Autodesk Inventor part; units mm, degrees
ref_plane "YZ Plane" through (0, 0, 0) normal (1, 0, 0) x (0, 1, 0)
ref_plane "XZ Plane" through (0, 0, 0) normal (0, 1, 0) x (-1, 0, 0)
ref_plane "XY Plane" through (0, 0, 0) normal (0, 0, 1) x (1, 0, 0)
sketch "Sketch1" plane through (0, 0, 0) normal (0, 0, 1) x (1, 0, 0)
  point P0 (0, 0)
sketch "Sketch2" plane through (0, 0, 0) normal (0, 0, 1) x (1, 0, 0)
  line L0 (20.0728, 0) -> (-15.1545, 0)
  line L1 (-19.19, 0) -> (-19.19, 50)
  line L2 (-19.19, 50) -> (70.81, 50)
  line L3 (70.81, 50) -> (70.81, 0)
  line L4 (70.81, 0) -> (-19.19, 0)
  line L5 (-19.19, 0) -> (-13.19, 0)
  line L6 (-13.19, 0) -> (-13.19, 15)
  point P0 (0, 0)
  dimension "d0" = 50
  dimension "d1" = 90
  dimension "d2" = 15
  dimension "d5" = 6
sketch "Sketch3" plane through (0, 0, 0) normal (0, 0, 1) x (1, 0, 0)
  line L0 (-13.1902, 15.9972) -> (-4.1902, 15.9972)
  line L1 (-4.1902, 15.9972) -> (-4.1902, 19.9972)
  line L2 (-4.1902, 19.9972) -> (-13.1902, 19.9972)
  line L3 (-13.1902, 19.9972) -> (-13.1902, 15.9972)
  line L4 (2.8098, 15.9972) -> (2.8098, 20.9972)
  line L5 (2.8098, 20.9972) -> (10.8098, 20.9972)
  line L6 (10.8098, 20.9972) -> (10.8098, 15.9972)
  line L7 (10.8098, 15.9972) -> (2.8098, 15.9972)
  line L8 (2.8098, 15.9972) -> (2.8098, 20.9972)
  line L9 (2.8098, 20.9972) -> (10.8098, 20.9972)
  line L10 (10.8098, 20.9972) -> (10.8098, 15.9972)
  line L11 (10.8098, 15.9972) -> (2.8098, 15.9972)
  line L12 (17.8096, 15.9972) -> (17.8096, 20.9972)
  line L13 (17.8096, 20.9972) -> (25.8096, 20.9972)
  line L14 (25.8096, 20.9972) -> (25.8096, 15.9972)
  line L15 (25.8096, 15.9972) -> (17.8096, 15.9972)
  line L16 (17.8096, 15.9972) -> (17.8096, 20.9972)
  line L17 (17.8096, 20.9972) -> (25.8096, 20.9972)
  line L18 (25.8096, 20.9972) -> (25.8096, 15.9972)
  line L19 (25.8096, 15.9972) -> (17.8096, 15.9972)
  circle A0 centre (36.289, 18.4972) radius 2.2825
  point P0 (0, 0)
  dimension "d7" = 9
  dimension "d8" = 4
  dimension "d9" = 9
  dimension "d11" = 5
  dimension "d12" = 8
  dimension "d13" = 5
  dimension "d14" = 8
  dimension "d16" = 7
  dimension "d18" = 5
  dimension "d19" = 8
  dimension "d20" = 5
  dimension "d21" = 8
  dimension "d22" = 5
  dimension "d23" = 8
  dimension "d24" = 5
  dimension "d25" = 8
  dimension "d27" = 5
  dimension "d28" = 8
  dimension "d29" = 5
  dimension "d30" = 8
sketch "Sketch4" plane through (0, 0, 0) normal (1, 0, 0) x (0, 1, 0)
  point P0 (0, 0)
sketch "Sketch5" plane through (0, 0, 0) normal (1, 0, 0) x (0, 1, 0)
  point P0 (0, 0)
sketch "Sketch6" plane through (0, 0, 0) normal (1, 0, 0) x (0, 1, 0)
  point P0 (0, 0)
extrude "Extrusion2" add sketch "Sketch2" against normal blind 210
sketch "Sketch7" plane through (70.81, 0, 0) normal (1, 0, 0) x (0, 0, -1)
  point P0 (0, 0)
sketch "Sketch8" plane through (-19.19, 50, 0) normal (0, 1, 0) x (1, 0, 0)
  point P0 (19.19, 0)
sketch "Sketch9" plane through (-19.19, 50, 0) normal (0, 1, 0) x (1, 0, 0)
  line L0 (0, 210) -> (90, 210)
  line L1 (0, 210) -> (3, 210)
  line L2 (3, 210) -> (0, 210)
  line L3 (90, 210) -> (87, 210)
  line L4 (90, 0) -> (0, 0)
  line L5 (90, 0) -> (90, 210)
  line L6 (90, 3) -> (90, 0)
  line L7 (0, 0) -> (0, 3)
  line L8 (0, 0) -> (0, 210)
  line L9 (3, 207) -> (87, 207)
  line L10 (87, 207) -> (87, 3)
  line L11 (87, 3) -> (3, 3)
  line L12 (3, 3) -> (3, 207)
  point P0 (19.19, 0)
  dimension "d39" = 3
  dimension "d40" = 3
extrude "Extrusion3" cut sketch "Sketch9" against normal blind 34.03 contours L9 L10 L11 L12
extrude "Extrusion4" cut sketch "Sketch3" against normal blind 33.25
sketch "Sketch10" plane through (0, 0, 0) normal (0, 0, 1) x (1, 0, 0)
  point P0 (0, 0)
sketch "Sketch11" plane through (0, 0, 0) normal (0, 0, 1) x (1, 0, 0)
  point P0 (0, 0)
sketch "Sketch12" plane through (67.81, 50, -3) normal (0, 0, -1) x (-1, 0, 0)
  point P0 (67.81, -50)
sketch "Sketch13" plane through (67.81, 50, -3) normal (0, 0, -1) x (-1, 0, 0)
  point P0 (67.81, -50)
sketch "Sketch14" plane through (0, 0, 0) normal (0, 0, 1) x (1, 0, 0)
  point P0 (0, 0)
sketch "Sketch15" plane through (70.81, 0, 0) normal (1, 0, 0) x (0, 0, -1)
  line L0 (0, 0) -> (0, 15)
  line L1 (0, 0) -> (0, 50)
  line L2 (0, 15) -> (1, 15)
  line L3 (1, 15) -> (15, 15)
  line L4 (15, 15) -> (15, 30)
  line L5 (15, 30) -> (1, 30)
  line L6 (1, 30) -> (1, 15)
  line L7 (15, 15) -> (19, 15)
  line L8 (19, 15) -> (33, 15)
  line L9 (33, 15) -> (33, 30)
  line L10 (33, 30) -> (19, 30)
  line L11 (19, 30) -> (19, 15)
  line L12 (33, 15) -> (37, 15)
  line L13 (37, 15) -> (52, 15)
  line L14 (52, 15) -> (52, 29)
  line L15 (52, 29) -> (37, 29)
  line L16 (37, 29) -> (37, 15)
  line L17 (52, 15) -> (58, 15)
  line L18 (58, 15) -> (63, 15)
  line L19 (63, 15) -> (63, 22)
  line L20 (63, 22) -> (58, 22)
  line L21 (58, 22) -> (58, 15)
  line L22 (63, 15) -> (83, 15)
  line L23 (83, 15) -> (91, 15)
  line L24 (91, 15) -> (91, 21)
  line L25 (91, 21) -> (83, 21)
  line L26 (83, 21) -> (83, 15)
  dimension "d53" = 15
  dimension "d54" = 1
  dimension "d55" = 14
  dimension "d56" = 15
  dimension "d57" = 4
  dimension "d58" = 14
  dimension "d59" = 15
  dimension "d60" = 4
  dimension "d61" = 15
  dimension "d62" = 14
  dimension "d63" = 6
  dimension "d64" = 5
  dimension "d65" = 7
  dimension "d66" = 20
  dimension "d67" = 8
  dimension "d68" = 6
extrude "Extrusion5" cut sketch "Sketch15" against normal blind 15.5
sketch "Sketch16" plane through (-19.19, 0, 0) normal (-1, 0, 0) x (0, 0, 1)
  line L0 (-3, 15.97) -> (-207, 15.97)
  line L1 (-134.7114, 15.97) -> (-93.0359, 15.97)
  line L2 (-93.0359, 15.97) -> (-93.0359, 28.1023)
  line L3 (-93.0359, 28.1023) -> (-134.7114, 28.1023)
  line L4 (-134.7114, 28.1023) -> (-134.7114, 15.97)
  point P0 (0, 0)
extrude "Extrusion6" cut sketch "Sketch16" against normal blind 14.25
properties part number "BOX_SAMPAH"
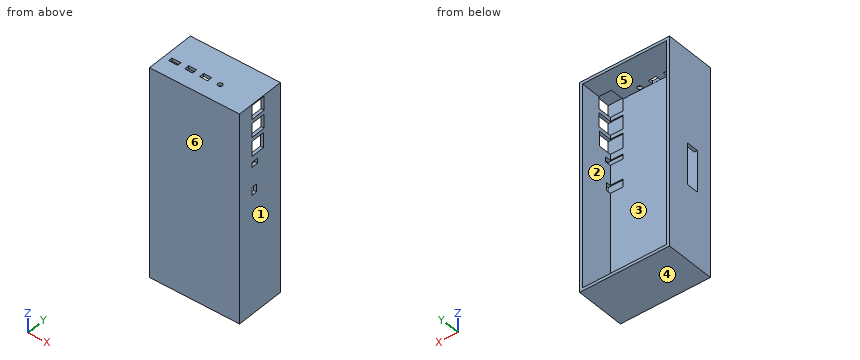
Can you work these out from the model? Positions are in its coordinate system, mm. Face numbers are marked on the shaded views. A direction names the side the tool comes from. Give positions to 0.01 mm unless a question says otherwise; leave off trailing zeros. Order: outer loops, then holes, each group sorted by start corner. A loop starts at its lowest first (then second) coordinate and runs counter-clockwise, first axis right, second up. Notation, with made-up numbers: (63, 75.25) - (83, 75.25) arc R24 cw to (83, 102.25) - close; hole circle Ø1 at (63.5, 25.5). An arc over 180 degrees is marked (long way). Use a Markdown table: item, result. Add a question column.
Q1. I'm going to push flat-ended pins straight in: pin 1 (2.5 mm diameter, centred on x = 65, z = -87, fed in from +Y); pin 2 (8 mm diameter, centred on x = -6.5, z = -181.5, fed in from +Y); pin 3 (0.8 mm diameter, centred on y = 15.5, z = -24, fed in from +X). Where does each tip first touch, or does it pass through?
Q2. Please list where these lines run through material, in increasing order: line 1 along Z through (x, y) = (56.5, 40); line 2 along X through (y, z) = (22.5, -177.5); line 3 along Z through (x, y) = (55.5, 21.5).
Q3. If we mould it in two halves opening along Z, with no side actions, what happens to the marked faces 3, 4, 5 and 6? For each: released by +Z, released by -Z, zero draft, split by the parting line, or undercut.
Q4. If we section it at B-B on y = 36.5: Write out the boundary of the cut face in (x, z), plus the area to 3 significant figures.
Q5. On a 3-axis mill with a long thin cutter (end or side, diameter ignored), from which of +Z, -Z, +X, -X, +Y, -Y can I reach the whole of each face in a straight line? I mean the marked faces 1 and 2. Say none if no direction works.
Q6. If we section it at C-C on z = -187.5: Write out the boundary of the cut face in (x, y), plus the area to 3 significant figures.
Q7. If we section it at A-A on z = -47: Write out the boundary of the cut face in (x, y).
Q8. If we section it at D-D on x = 53: Write out the boundary of the cut face in (y, z).
Answers follow:
| question | item | result |
|---|---|---|
| 1 | pin 1 | stops at y = 15 |
| 1 | pin 2 | stops at y = 15.97 |
| 1 | pin 3 | stops at x = 55.31 |
| 2 | line 1 | z = -210 to -207, -3 to 0 |
| 2 | line 2 | x = -19.19 to -16.19, 67.81 to 70.81 |
| 2 | line 3 | z = -210 to -207, -1 to 0 |
| 3 | face 3 | undercut |
| 3 | face 4 | released by -Z |
| 3 | face 5 | undercut |
| 3 | face 6 | zero draft |
| 4 | outline | (-19.19, -210) - (70.81, -210) - (70.81, 0) - (-19.19, 0) - close; hole (-16.19, -207) - (67.81, -207) - (67.81, -3) - (-16.19, -3) - close |
| 4 | area | 1,760 mm^2 |
| 5 | face 1 | +Z, -Z, +X, +Y, -Y |
| 5 | face 2 | +Y |
| 6 | outline | (-19.19, 0) - (70.81, 0) - (70.81, 50) - (67.81, 50) - (67.81, 15.97) - (-16.19, 15.97) - (-16.19, 50) - (-19.19, 50) - close |
| 6 | area | 1,640 mm^2 |
| 7 | outline | (-19.19, 0) - (70.81, 0) - (70.81, 15) - (55.31, 15) - (55.31, 15.97) - (-16.19, 15.97) - (-16.19, 50) - (-19.19, 50) - close; (67.81, 29) - (70.81, 29) - (70.81, 50) - (67.81, 50) - close |
| 8 | outline | (0, -210) - (50, -210) - (50, -207) - (15.97, -207) - (15.97, -3) - (50, -3) - (50, 0) - (0, 0) - close |
